Work out the finished part from the listing and answer in its coordinate system (mm). A direction names the side the tool comes from. Coordinates: 2 decimals unless noted, no trailing zeros. Order: outer loops, then holes, each group sorted by start corner. A loop starts at its lowest first (then second) coordinate and runs counter-clockwise, first axis right, second up. Notation, with made-up numbers: M 22,61.5 L 70,61.5 A31 cw 70,99.5 Z; hole C -22.5,5 d1. An arc over 180 degrees is marked long. Use a Markdown table: item, result.
from build123d import *

# Parameters (mm, degrees)
SKETCH1_R           = 2.9
BOSS_EXTRUDE1_DEPTH = 30
CUT_EXTRUDE1_DEPTH  = 5.5
SKETCH3_R           = 1.5
CUT_EXTRUDE2_DEPTH  = 31.45931713
FILLET1_R           = 1.25
FILLET2_R           = 0.25


with BuildPart() as part:
    # Sketch1 → Boss-Extrude1 (new body)
    with BuildSketch(Plane.XY):
        Circle(SKETCH1_R)
    extrude(amount=BOSS_EXTRUDE1_DEPTH)

    # Sketch2 → Cut-Extrude1 (cut)
    with BuildSketch(Plane(origin=(0, 0, 0), x_dir=(-1, 0, 0), z_dir=(0, 0, -1))):
        with BuildLine():
            Line((-1.5, -2.481934729), (-1.5, 2.481934729))
            ThreePointArc((-1.5, 2.481934729), (-2.9, 0), (-1.5, -2.481934729))
        make_face()
        with BuildLine():
            ThreePointArc((2.9, 0), (2.525866188, 1.424780685), (1.5, 2.481934729))
            Line((1.5, 2.481934729), (1.5, -2.481934729))
            ThreePointArc((1.5, -2.481934729), (2.525866188, -1.424780685), (2.9, 0))
        make_face()
    extrude(amount=-CUT_EXTRUDE1_DEPTH, mode=Mode.SUBTRACT)

    # Sketch3 → Cut-Extrude2 (cut, through all)
    with BuildSketch(Plane.ZY.offset(1.5)):
        with Locations((2.75, 0)):
            Circle(SKETCH3_R)
    extrude(amount=-CUT_EXTRUDE2_DEPTH, mode=Mode.SUBTRACT)

    # Fillet1
    fillet1_edges = [part.edges().sort_by_distance(p)[0] for p in [
        (0, 2.9, 0),
        (0, -2.9, 0),
    ]]
    fillet(fillet1_edges, radius=FILLET1_R)

    # Fillet2
    fillet2_edges = [part.edges().sort_by_distance(p)[0] for p in [
        (1.5, 0, 5.5),
        (-1.5, 0, 5.5),
    ]]
    fillet(fillet2_edges, radius=FILLET2_R)


solid = part.part
(1) Determine the mould class of faces 1 (the cylindrical face through (1.34, -2.57, 15.42)), 2 (the cylindrical face through (-0.021, -0.575, 4.136)), 3 (the flat face through (-2, 0, 5.5)) for opening direction Y: pulls with the +Y half, pulls with the -Y half, needs draft (parallel to the pull), parting line crosses it, or undercut.
Conclusion:
| item | result |
|---|---|
| face 1 | parting line crosses it |
| face 2 | undercut |
| face 3 | needs draft |
(2) Straight lines are drawn through the part: L1, parallel to Z at x = -1.9, y = 1.35; L2, parallel to Y at x = -0.55, z = 2.75; L3, parallel to Y at x = -0.15, z = 12. For each, find the intervals that lie inside material, in ascending order.
Conclusion:
| item | result |
|---|---|
| L1 | 5.5 to 30 |
| L2 | -2.85 to -1.5, 1.5 to 2.85 |
| L3 | -2.9 to 2.9 |
(3) Given P1, Ø0.6, axis at x = -2.5, y = -0.5, coming from the -Z side, flat-ended and moving along its own axis, determine where the tip first touches the part or whether it passes through.
Conclusion:
| item | result |
|---|---|
| P1 | z = 5.5 |
(4) A cutting plane is placed at B-B (y = 0). Determine the outline of the cut face in (x, z).
Conclusion:
| item | result |
|---|---|
| outline | M -2.9,5.5 L -1.75,5.5 A0.25 cw -1.5,5.25 L -1.5,4.25 L 1.5,4.25 L 1.5,5.25 A0.25 cw 1.75,5.5 L 2.9,5.5 L 2.9,30 L -2.9,30 Z; M -1.5,0 L 1.5,0 L 1.5,1.25 L -1.5,1.25 Z |
(5) A cutting plane is placed at A-A (z = 2.75). Determine the outline of the cut face in (x, y).
Conclusion:
| item | result |
|---|---|
| outline | M -1.5,-2.48 A2.9 ccw 1.5,-2.48 L 1.5,-1.5 L -1.5,-1.5 Z; M -1.5,1.5 L 1.5,1.5 L 1.5,2.48 A2.9 ccw -1.5,2.48 Z |
(6) Which of the six approach directions +Z, -Z, +X, -X, +Y, -Y give full straight-line access (tool end or side, diameter ignored) to faces 4 (the flat face through (2, 0, 5.5)), 5 (the flat face through (0, 0, 0)), 6 (the flat face through (-1.5, 2, 3))?
Conclusion:
| item | result |
|---|---|
| face 4 | -Z, +X, +Y, -Y |
| face 5 | -Z, +X, -X, +Y, -Y |
| face 6 | -Z, -X, +Y, -Y |
(7) A cutting plane is placed at D-D (x = 2.1). Determine the outline of the cut face in (y, z).
Conclusion:
| item | result |
|---|---|
| outline | M -2,5.5 L 2,5.5 L 2,30 L -2,30 Z |
(8) A cutting plane is placed at C-C (x = 0). Determine the outline of the cut face in (y, z).
Conclusion:
| item | result |
|---|---|
| outline | M -2.9,1.25 A1.25 ccw -1.65,0 L 1.65,0 A1.25 ccw 2.9,1.25 L 2.9,30 L -2.9,30 Z; hole C 0,2.75 d3 |
